The model under review builds one solid part; all positions refer to its coordinate system, in mm. A direction names the side the tool comes from. Coordinates: 2 decimals unless noted, no trailing zeros. Write each loop counter-clockwise with the first axis right and the second up, starting at its lowest first coordinate (ties: lowest second). Pieces come first, ordered by that corner, then holes.
```python
from build123d import *

# Parameters (mm, degrees)
F0_R     = 2.9240242171
F1_DEPTH = 25.4


with BuildPart() as f1:
    # F0 (on Front) → F1 (new body)
    with BuildSketch(Plane.XZ):
        with BuildLine():
            ThreePointArc((-9.5175899986, 89.6733759373), (-6.601047317, 83.1822994355), (0, 80.5240162142))
            ThreePointArc((0, 80.5240162142), (6.7351920908, 83.3138241234), (9.525, 90.0490162142))
            ThreePointArc((9.525, 90.0490162142), (9.5063048942, 90.6454994562), (9.4502929642, 91.2396412142))
            ThreePointArc((9.4502929642, 91.2396412142), (-0.7838551857, 99.5417079319), (-9.5175899986, 89.6733759373))
        make_face()
        with BuildLine():
            ThreePointArc((3.175, 90.0490162142), (2.2450640303, 87.8039521839), (0, 86.8740162142))
            ThreePointArc((0, 86.8740162142), (-2.2450640303, 92.2940802445), (3.175, 90.0490162142))
        make_face(mode=Mode.SUBTRACT)
        with BuildLine():
            ThreePointArc((9.525, 90.0490162142), (6.7351920908, 83.3138241234), (0, 80.5240162142))
            Line((0, 80.5240162142), (0, 55.1240162142))
            ThreePointArc((0, 55.1240162142), (10.5003255158, 51.1552662142), (15.7504882737, 41.2333912142))
            Line((15.7504882737, 41.2333912142), (9.4502929642, 91.2396412142))
            ThreePointArc((9.4502929642, 91.2396412142), (9.5063048942, 90.6454994562), (9.525, 90.0490162142))
        make_face()
        with BuildLine():
            Line((0, 55.1240162142), (0, 80.5240162142))
            ThreePointArc((0, 80.5240162142), (-6.601047317, 83.1822994355), (-9.5175899986, 89.6733759373))
            Line((-9.5175899986, 89.6733759373), (-15.7451890335, 41.2750091314))
            ThreePointArc((-15.7451890335, 41.2750091314), (-10.4845836217, 51.1691307808), (0, 55.1240162142))
        make_face()
        with Locations((-7.9077519476, 77.4001702666)):
            Circle(F0_R, mode=Mode.SUBTRACT)
        with BuildLine():
            ThreePointArc((15.7504882737, 41.2333912142), (10.5003255158, 51.1552662142), (0, 55.1240162142))
            Line((0, 55.1240162142), (0, 42.4240162142))
            ThreePointArc((0, 42.4240162142), (2.2450640303, 41.4940802445), (3.175, 39.2490162142))
            ThreePointArc((3.175, 39.2490162142), (2.2450640303, 37.0039521839), (0, 36.0740162142))
            Line((0, 36.0740162142), (0, 23.3740162142))
            ThreePointArc((0, 23.3740162142), (10.6492737428, 27.4758011159), (15.7954255641, 37.6615162142))
            ThreePointArc((15.7954255641, 37.6615162142), (15.8550939106, 38.4542696601), (15.875, 39.2490162142))
            ThreePointArc((15.875, 39.2490162142), (15.8438414904, 40.2431549508), (15.7504882737, 41.2333912142))
        make_face()
        with BuildLine():
            Line((0, 42.4240162142), (0, 55.1240162142))
            ThreePointArc((0, 55.1240162142), (-10.4845836217, 51.1691307808), (-15.7451890335, 41.2750091314))
            ThreePointArc((-15.7451890335, 41.2750091314), (-11.9201145666, 28.7644325925), (0, 23.3740162142))
            Line((0, 23.3740162142), (0, 36.0740162142))
            ThreePointArc((0, 36.0740162142), (-3.175, 39.2490162142), (0, 42.4240162142))
        make_face()
        with BuildLine():
            ThreePointArc((0, 23.3740162142), (-11.9201145666, 28.7644325925), (-15.7451890335, 41.2750091314))
            Line((-15.7451890335, 41.2750091314), (-16.2073878987, 37.6829875368))
            Line((-16.2073878987, 37.6829875368), (-9.4709206869, -25.2645351372))
            ThreePointArc((-9.4709206869, -25.2645351372), (-7.0844795723, -17.8842126898), (0, -14.7259837858))
            Line((0, -14.7259837858), (0, 23.3740162142))
        make_face()
        with BuildLine():
            ThreePointArc((15.7954255641, 37.6615162142), (10.6492737428, 27.4758011159), (0, 23.3740162142))
            Line((0, 23.3740162142), (0, -14.7259837858))
            ThreePointArc((0, -14.7259837858), (6.7351920908, -17.515791695), (9.525, -24.2509837858))
            Line((9.525, -24.2509837858), (36.5125, -24.2509837858))
            ThreePointArc((36.5125, -24.2509837858), (38.8373399243, -18.6383237101), (44.45, -16.3134837858))
            Line((44.45, -16.3134837858), (18.9672152943, -15.403384332))
            ThreePointArc((18.9672152943, -15.403384332), (13.2606937919, -12.6853206287), (11.3406209777, -6.6632297674))
            Line((11.3406209777, -6.6632297674), (15.7954255641, 37.6615162142))
        make_face()
        with BuildLine():
            Line((0, -21.0759837858), (0, -14.7259837858))
            ThreePointArc((0, -14.7259837858), (-7.0844795723, -17.8842126898), (-9.4709206869, -25.2645351372))
            ThreePointArc((-9.4709206869, -25.2645351372), (-6.366771096, -31.3354633582), (0, -33.7759837858))
            Line((0, -33.7759837858), (0.6773435479, -33.7518695718))
            ThreePointArc((0.6773435479, -33.7518695718), (6.9705567315, -30.7422828741), (9.525, -24.2509837858))
            Line((9.525, -24.2509837858), (3.175, -24.2509837858))
            ThreePointArc((3.175, -24.2509837858), (-2.2450640303, -26.4960478161), (0, -21.0759837858))
        make_face()
        with BuildLine():
            Line((36.5125, -24.2509837858), (9.525, -24.2509837858))
            ThreePointArc((9.525, -24.2509837858), (6.9705567315, -30.7422828741), (0.6773435479, -33.7518695718))
            Line((0.6773435479, -33.7518695718), (44.7324052746, -32.1834584004))
            ThreePointArc((44.7324052746, -32.1834584004), (38.9380895153, -29.9626165697), (36.5125, -24.2509837858))
        make_face()
        with BuildLine():
            Line((0.6773435479, -33.7518695718), (0, -33.7759837858))
            ThreePointArc((0, -33.7759837858), (0.3388863295, -33.7699533233), (0.6773435479, -33.7518695718))
        make_face()
        with BuildLine():
            ThreePointArc((44.45, -16.3134837858), (38.8373399243, -18.6383237101), (36.5125, -24.2509837858))
            ThreePointArc((36.5125, -24.2509837858), (38.9380895153, -29.9626165697), (44.7324052746, -32.1834584004))
            ThreePointArc((44.7324052746, -32.1834584004), (50.1616327839, -29.7628942705), (52.3875, -24.2509837858))
            ThreePointArc((52.3875, -24.2509837858), (50.0626600757, -18.6383237101), (44.45, -16.3134837858))
        make_face()
        with BuildLine():
            ThreePointArc((47.625, -24.2509837858), (44.45, -27.4259837858), (41.275, -24.2509837858))
            ThreePointArc((41.275, -24.2509837858), (44.45, -21.0759837858), (47.625, -24.2509837858))
        make_face(mode=Mode.SUBTRACT)
        with BuildLine():
            ThreePointArc((9.525, -24.2509837858), (6.7351920908, -17.515791695), (0, -14.7259837858))
            Line((0, -14.7259837858), (0, -21.0759837858))
            ThreePointArc((0, -21.0759837858), (2.2450640303, -22.0059197555), (3.175, -24.2509837858))
            Line((3.175, -24.2509837858), (9.525, -24.2509837858))
        make_face()
    extrude(amount=F1_DEPTH)


solid = f1.part
```
Item 1: Take a section at C-C, the plane x = 31. Write out the cut boundary in (y, z), plus the area to 3 significant figures.
Solved:
outline: (-25.4, -32.67) - (0, -32.67) - (0, -15.83) - (-25.4, -15.83) - close
area: 428 mm2
Item 2: Machinability: for faces 4 (the face through (13.537, -12.522, 15.189)), 5 (the face through (2, 0, 19)), which of the approach directions +Z, -Z, +X, -X, +Y, -Y give a long, thin tool a straight path to every point of the face, cutting with its end or side? Answer none if there is none.
Solved:
face 4: +X, +Y, -Y
face 5: +Z, -Z, +X, -X, +Y
Item 3: Take a section at A-A, the plane y = -17.5. Count the separate pieces of the cut face and the enclosed holes in it, plus the area to 3 significant figures.
Solved:
separate pieces: 1
enclosed holes: 5
area: 3,790 mm2
Item 4: For pin 1 (6 mm diameter, centred on y = -12, z = 18, fed in from -X); pin 2 (4 mm diameter, centred on x = 35, y = -19, fed in from +Z); pin 3 (5.5 mm diameter, centred on x = 0, z = -24.25, fed in from +Y); pin 4 (10 mm diameter, centred on x = 0, z = 90.05, fed in from +Y), all flat-tipped, find the tip position at first contact; note any pin that passes through.
Solved:
pin 1: stops at x = -14.42
pin 2: stops at z = -15.9
pin 3: passes through
pin 4: stops at y = 0
Item 5: Mouldability with a two-part tool opening along Z and no side actions: class faces 1 (the face through (52.387, -12.522, -24.282)), 2 (the face through (-12.886, -12.522, 6.65)), 3 (the face through (-8.542, -12.522, 74.546)) as pulls with the +Z half, pulls with the -Z half, needs draft (parallel to the pull), parting line crosses it, or undercut.
Solved:
face 1: parting line crosses it
face 2: pulls with the -Z half
face 3: undercut
Item 6: To check wall thickness, follow line 1 along X through (y, z) = (-13.5, -24); line 2 along Z through (x, y) = (-2.5, -2); line 3 along X through (y, z) = (-7, 39). State the ranges of each line that lie inside material, in increasing order.
Solved:
line 1: x = -9.61 to -3.17, 3.17 to 41.28, 47.62 to 52.38
line 2: z = -33.44 to -26.21, -22.29 to 37.29, 41.21 to 88.09, 92.01 to 99.24
line 3: x = -16.04 to -3.17, 3.17 to 15.87
Item 7: Take a section at B-B, the plane z = 66.5. Write out the cut boundary in (x, y), plus the area to 3 significant figures.
Solved:
outline: (-12.5, -25.4) - (12.57, -25.4) - (12.57, 0) - (-12.5, 0) - close
area: 637 mm2
